Verification items for the finished model (mm, model axes). Face numbers are marked on the shaded views. A direction names the side the tool comes from. Give positions to 0.01 mm unless a question says otherwise; leave off trailing zeros. Loops run counter-clockwise (first coordinate to the right, second up) from the corner with the lowest first, then second, coordinate; pieces in that order, holes last. Notation, with made-up numbers: (74.25, 73) - (121.25, 73) arc R32 cw to (121.25, 111) - close; hole circle Ø2 at (4.5, 44). An arc over 180 degrees is marked (long way). Put each result on its own line as item: value. Start each with the question number.
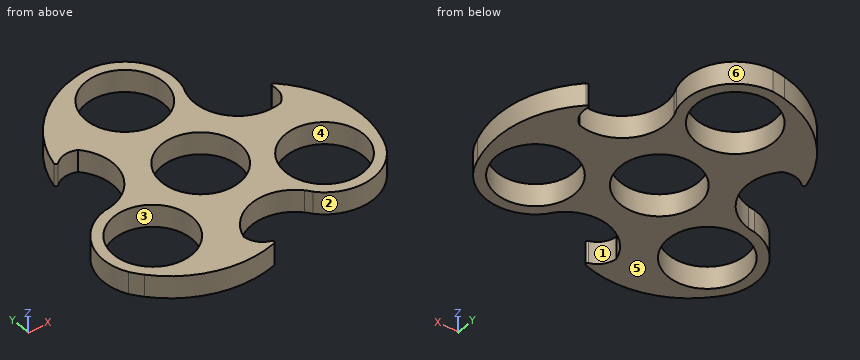
```python
from build123d import *

# Parameters (mm, degrees)
F0_R     = 11.05
F1_DEPTH = 6.35
F2_R     = 0.508


# Not quite as in the source:
# - a feature names something its author has since deleted; it is built from what else it names


with BuildPart() as f1:
    # F0 (on Top) → F1 (new body)
    with BuildSketch(Plane.XY):
        with BuildLine():
            ThreePointArc((27.1429276567, 6.1352837814), (15.2810658667, 9.7013912391), (12.5387063316, 21.7803130331))
            ThreePointArc((12.5387063316, 21.7803130331), (12.8751071514, 22.7165186649), (13.2860771432, 23.6224712919))
            ThreePointArc((13.2860771432, 23.6224712919), (11.3021408603, 36.1511212373), (0, 41.91))
            ThreePointArc((0, 41.91), (-1.8008358417, 41.7320810261), (-3.5869805559, 41.4416469548))
            ThreePointArc((-3.5869805559, 41.4416469548), (-18.8414291839, 33.1449919843), (-26.5736300498, 17.5968166441))
            ThreePointArc((-26.5736300498, 17.5968166441), (-23.32919107, 20.6410473634), (-18.8847754424, 20.4388229931))
            ThreePointArc((-18.8847754424, 20.4388229931), (-16.0421841985, 8.3830956179), (-25.1316575548, -0.0313183028))
            ThreePointArc((-25.1316575548, -0.0313183028), (-26.1106358251, -0.2080894629), (-27.1006988106, -0.3051553233))
            ThreePointArc((-27.1006988106, -0.3051553233), (-36.958859797, -8.2876195165), (-36.2951246726, -20.955))
            ThreePointArc((-36.2951246726, -20.955), (-35.2406244005, -22.4256101), (-34.0960287596, -23.8272397617))
            ThreePointArc((-34.0960287596, -23.8272397617), (-19.2836904747, -32.889652309), (-1.9524752146, -31.811847016))
            ThreePointArc((-1.9524752146, -31.811847016), (-6.2110758425, -30.5241957981), (-8.2581522143, -26.5741067745))
            ThreePointArc((-8.2581522143, -26.5741067745), (0.7611183318, -18.0844868571), (12.5929512232, -21.7489947303))
            ThreePointArc((12.5929512232, -21.7489947303), (13.2355286736, -22.508429202), (13.8146216674, -23.3173159686))
            ThreePointArc((13.8146216674, -23.3173159686), (25.6567189367, -27.8635017208), (36.2951246726, -20.955))
            ThreePointArc((36.2951246726, -20.955), (37.0414602422, -19.3064709261), (37.6830093155, -17.6144071931))
            ThreePointArc((37.6830093155, -17.6144071931), (38.1251196586, -0.2553396753), (28.5261052644, 14.2150303719))
            ThreePointArc((28.5261052644, 14.2150303719), (29.5402669125, 9.8831484346), (27.1429276567, 6.1352837814))
        make_face()
        with Locations((-24.1967497817, -13.97)):
            Circle(F0_R, mode=Mode.SUBTRACT)
        Circle(F0_R, mode=Mode.SUBTRACT)
        with Locations((24.1967497817, -13.97)):
            Circle(F0_R, mode=Mode.SUBTRACT)
        with Locations((0, 27.94)):
            Circle(F0_R, mode=Mode.SUBTRACT)
    extrude(amount=F1_DEPTH)

    # F2
    f2_edges = [f1.edges().sort_by_distance(p)[0] for p in [
        (-1.952475, -31.811847, 3.175),
        (-26.57363, 17.596817, 3.175),
        (28.526105, 14.21503, 3.175),
    ]]
    fillet(f2_edges, radius=F2_R)


solid = f1.part
```
1) Section check C-C, the plane x = 1.5. Enter the section's corners in (y, z).
2) Section check A-A, the plane y = -2. Enter the section's corners in (x, z).
3) Set-up check for the marked faces 1 and 2: record each of +Z, -Z, +X, -X, +Y, -Y from which the full face is reachable in a straight line by a thin tool's end or side.
4) Draft check along X on the marked faces 3, 4, 5 and 6. Enter one of: pulls with the +X half, pulls with the -X half, needs draft (parallel to the pull), parting line crosses it, or undercut.
5) Section check B-B, the plane x = -32.5. Enter the section's corners in (y, z).
6) Section check D-D, the plane z = 4.25. State how many separate pieces and enclosed holes the cut face has, plus the area to 3 significant figures.
7) Depth check by flat-ended pin: P1, Ø1, axis at y = 21, z = 3.5, coming from the -X side; P2, Ø12, axis at x = -3, y = -3.5, coming from the +Z side; P3, Ø4, axis at x = 30.5, y = -24, coming from the -Z side. Enter the tip coordinate at first touch or a pass-through.
8) Scan lines: line 1 along Y through (x, z) = (-24, 4.5); line 2 along X through (y, z) = (35, 6); line 3 along Y through (x, z) = (26.5, 4). Record each from-to range of solid material in increasing order. Write a range as from..to.
Results are:
1. outline: (-17.94, 0) - (-10.95, 0) - (-10.95, 6.35) - (-17.94, 6.35) - close; (10.95, 0) - (16.99, 0) - (16.99, 6.35) - (10.95, 6.35) - close; (38.89, 0) - (41.83, 0) - (41.83, 6.35) - (38.89, 6.35) - close
2. outline: (-31.4, 0) - (-10.87, 0) - (-10.87, 6.35) - (-31.4, 6.35) - close; (10.87, 0) - (38.57, 0) - (38.57, 6.35) - (10.87, 6.35) - close
3. face 1: +Z, -Z
3. face 2: +Z, -Z, -Y
4. face 3: undercut
4. face 4: undercut
4. face 5: needs draft
4. face 6: pulls with the +X half
5. outline: (-25.52, 0) - (-21.26, 0) - (-21.26, 6.35) - (-25.52, 6.35) - close; (-6.68, 0) - (-2.74, 0) - (-2.74, 6.35) - (-6.68, 6.35) - close
6. separate pieces: 1
6. enclosed holes: 4
6. area: 1,860 mm2
7. P1: stops at x = -25.96
7. P2: passes through
7. P3: stops at z = 0
8. line 1: y = -31.27..-25.02, -2.92..0.28, 20.34..25.77
8. line 2: x = -16.88..-8.5, 8.5..12.05
8. line 3: y = -27.75..-24.78, -3.16..6
